```python
from build123d import *

# Parameters (mm, degrees)
BOSS_EXTRUDE1_DEPTH = 5
BOSS_EXTRUDE2_DEPTH = 80
SKETCH4_W           = 56.5
SKETCH4_H           = 56.2
SKETCH4_R           = 19.25
SKETCH4_R_2         = 2.5
BOSS_EXTRUDE3_DEPTH = 8
BOSS_EXTRUDE4_DEPTH = 3


with BuildPart() as part:
    # Sketch2 → Boss-Extrude1 (new body)
    with BuildSketch(Plane(origin=(0, 0, 0), x_dir=(1, 0, 0), z_dir=(0, 1, 0))):
        with BuildLine():
            Line((-30, -35), (30, -35))
            ThreePointArc((30, -35), (33.535533906, -33.535533906), (35, -30))
            Line((35, -30), (35, 30))
            ThreePointArc((35, 30), (33.535533906, 33.535533906), (30, 35))
            Line((30, 35), (-30, 35))
            ThreePointArc((-30, 35), (-33.535533906, 33.535533906), (-35, 30))
            Line((-35, 30), (-35, -30))
            ThreePointArc((-35, -30), (-33.535533906, -33.535533906), (-30, -35))
        make_face()
    boss_extrude1 = extrude(amount=BOSS_EXTRUDE1_DEPTH)

    # Sketch3 → Boss-Extrude2 (add)
    with BuildSketch(Plane(origin=(0, 5, 0), x_dir=(1, 0, 0), z_dir=(0, 1, 0))):
        Polygon((-2.5, 2.5), (-2.5, 35), (2.5, 35), (2.5, 2.5), (35, 2.5), (35, -2.5), (2.5, -2.5), (2.5, -35), (-2.5, -35), (-2.5, -2.5), (-35, -2.5), (-35, 2.5), align=None)
    extrude(amount=BOSS_EXTRUDE2_DEPTH)

    # Mirror1: Boss-Extrude1 across plane
    add(boss_extrude1.mirror(Plane.ZX.offset(45)))

    # Sketch4 → Boss-Extrude3 (add)
    with BuildSketch(Plane(origin=(35, 0, 0), x_dir=(0, 0, -1), z_dir=(1, 0, 0))):
        with Locations((0, 118.1)):
            Rectangle(SKETCH4_W, SKETCH4_H)
        with Locations((0, 118.1)):
            Circle(SKETCH4_R, mode=Mode.SUBTRACT)
        with Locations((-23.829498526, 141.929498526)):
            Circle(SKETCH4_R_2, mode=Mode.SUBTRACT)
        with Locations(Location((23.829498526, 141.929498526, 0), (0, 0, 180))):
            Circle(SKETCH4_R_2, mode=Mode.SUBTRACT)
        with Locations((23.829498526, 94.270501474)):
            Circle(SKETCH4_R_2, mode=Mode.SUBTRACT)
        with Locations(Location((-23.829498526, 94.270501474, 0), (0, 0, 180))):
            Circle(SKETCH4_R_2, mode=Mode.SUBTRACT)
    extrude(amount=-BOSS_EXTRUDE3_DEPTH)

    # Sketch5 → Boss-Extrude4 (add)
    with BuildSketch(Plane.XY.offset(28.25)):
        Polygon((35, 90), (-30, 90), (27, 146.2), (35, 146.2), align=None)
    boss_extrude4 = extrude(amount=BOSS_EXTRUDE4_DEPTH)

    # Mirror2: Boss-Extrude4 across plane
    add(boss_extrude4.mirror(Plane(origin=(0, 0, 0), x_dir=(1, 0, 0), z_dir=(0, 0, -1))))


solid = part.part
```
Model file for the job. Use its own axes, mm. A direction names the side the tool comes from. Give positions to 0.01 mm unless a question says otherwise; leave off trailing zeros. Write each loop counter-clockwise with the first axis right and the second up, starting at its lowest first coordinate (ties: lowest second). Pieces come first, ordered by that corner, then holes. Notation, with made-up numbers: M -22,64 L 35,64 A29 cw 35,85 Z; hole C 35.5,23 d4. An arc over 180 degrees is marked long. Use a Markdown table: item, result.
1) Cut at D-D (z = 11). List the corners of the cut face in (x, y).
Responses:
| item | result |
|---|---|
| outline | M -35,0 L 35,0 L 35,5 L 2.5,5 L 2.5,85 L 35,85 L 35,102.3 L 27,102.3 L 27,90 L -35,90 L -35,85 L -2.5,85 L -2.5,5 L -35,5 Z; M 27,133.9 L 35,133.9 L 35,146.2 L 27,146.2 Z |
2) Tool access for faces 5 (the flat face through (-19, 5, -19)), 6 (the flat face through (12, 106, 28.25)), 7 (the flat face through (-19, 5, 19)), 8 (the flat face through (19, 44, 2.5)): list every direction of +Z, -Z, +X, -X, +Y, -Y with a clear straight run to the whole face (end or side of a thin tool).
Responses:
| item | result |
|---|---|
| face 5 | -Z, -X |
| face 6 | -X, +Y |
| face 7 | +Z, -X |
| face 8 | +Z, +X |
3) Cut at A-A (z = 0). List the corners of the cut face in (x, y).
Responses:
| item | result |
|---|---|
| outline | M -35,0 L 35,0 L 35,98.85 L 27,98.85 L 27,90 L -35,90 Z; M 27,137.35 L 35,137.35 L 35,146.2 L 27,146.2 Z |
4) Drill centre lines: line 1 (Y direction, x = 31.5, z = 29.5); line 2 (Y direction, x = 26, z = 13); line 3 (Z direction, x = -3.5, y = 107). Where is each one in solid material? Low to high. Write a range as from..to.
Responses:
| item | result |
|---|---|
| line 1 | y = 0..5, 85..146.2 |
| line 2 | y = 0..5, 85..90 |
| line 3 | z = -31.25..-28.25, 28.25..31.25 |
5) Pull direction Z, two halves, no side cores. Call faces 1 (the flat face through (-1, 90, 0)), 2 (the cylindrical face through (34, 88, -33)), 3 (the flat face through (31, 146.2, 0)), 4 (the cylindrical face through (31.06, 139.49, 24.37)): +Z half, -Z half, draft (parallel to the pull), parting line (faces both ways), or undercut.
Responses:
| item | result |
|---|---|
| face 1 | undercut |
| face 2 | -Z half |
| face 3 | draft |
| face 4 | undercut |
6) Cut at C-C (y = 62.5). List the corners of the cut face in (x, z).
Responses:
| item | result |
|---|---|
| outline | M -35,-2.5 L -2.5,-2.5 L -2.5,-35 L 2.5,-35 L 2.5,-2.5 L 35,-2.5 L 35,2.5 L 2.5,2.5 L 2.5,35 L -2.5,35 L -2.5,2.5 L -35,2.5 Z |
7) Pin check, flat tips, straight feed: pin 1 (6 mm diameter, centred on x = -22, z = 21.5, fed in from +Y); pin 2 (5 mm diameter, centred on y = 30.5, z = -13, fed in from -X); pin 3 (1.5 mm diameter, centred on x = 8, y = 36.5, fed in from -Z). Stop position of each tip, or through.
Responses:
| item | result |
|---|---|
| pin 1 | stops at y = 90 |
| pin 2 | stops at x = -2.5 |
| pin 3 | stops at z = -2.5 |
8) Cut at B-B (y = 118.1). List the corners of the cut face in (x, z).
Responses:
| item | result |
|---|---|
| outline | M -1.5,-31.25 L 35,-31.25 L 35,-19.25 L 27,-19.25 L 27,-28.25 L -1.5,-28.25 Z; M -1.5,28.25 L 27,28.25 L 27,19.25 L 35,19.25 L 35,31.25 L -1.5,31.25 Z |
